```python
from build123d import *

# Parameters (mm, degrees)
SKETCH2_W             = 25
SKETCH2_H             = 25
BOSS_EXTRUDE1_DEPTH   = 760
BOSS_EXTRUDE1_2_DEPTH = 760
BOSS_EXTRUDE1_3_DEPTH = 760
BOSS_EXTRUDE1_4_DEPTH = 760
SKETCH3_W             = 25
SKETCH3_H             = 25
BOSS_EXTRUDE2_DEPTH   = 470
SKETCH6_W             = 25
SKETCH6_H             = 25
BOSS_EXTRUDE4_DEPTH   = 675
SKETCH10_W            = 25
SKETCH10_H            = 25
BOSS_EXTRUDE5_DEPTH   = 470
SKETCH11_W            = 25
SKETCH11_H            = 50
BOSS_EXTRUDE6_DEPTH   = 470
SKETCH12_R            = 650
BOSS_EXTRUDE7_DEPTH   = 20
SKETCH13_R            = 25
CUT_EXTRUDE3_DEPTH    = 20


with BuildPart() as part:
    # Sketch2 → Boss-Extrude1 (new body)
    with BuildSketch(Plane(origin=(0, 0, 0), x_dir=(1, 0, 0), z_dir=(0, 1, 0))):
        with Locations((-66.268467475, 428.678343046)):
            Rectangle(SKETCH2_W, SKETCH2_H)
    extrude(amount=-BOSS_EXTRUDE1_DEPTH)



with BuildPart() as body_2:
    # Sketch2 → Boss-Extrude1 2 (new body)
    with BuildSketch(Plane(origin=(0, 0, 0), x_dir=(1, 0, 0), z_dir=(0, 1, 0))):
        with Locations((628.731532525, 428.678343046)):
            Rectangle(SKETCH2_W, SKETCH2_H)
    extrude(amount=-BOSS_EXTRUDE1_2_DEPTH)


with BuildPart() as body_3:
    # Sketch2 → Boss-Extrude1 3 (new body)
    with BuildSketch(Plane(origin=(0, 0, 0), x_dir=(1, 0, 0), z_dir=(0, 1, 0))):
        with Locations((628.731532525, -61.321656954)):
            Rectangle(SKETCH2_W, SKETCH2_H)
    extrude(amount=-BOSS_EXTRUDE1_3_DEPTH)


with BuildPart() as body_4:
    # Sketch2 → Boss-Extrude1 4 (new body)
    with BuildSketch(Plane(origin=(0, 0, 0), x_dir=(1, 0, 0), z_dir=(0, 1, 0))):
        with Locations((-66.268467475, -61.321656954)):
            Rectangle(SKETCH2_W, SKETCH2_H)
    extrude(amount=-BOSS_EXTRUDE1_4_DEPTH)


with BuildPart() as part_1:
    add(part.part)

    add(body_2.part)  # Boss-Extrude2 merges body 2

    add(body_3.part)  # Boss-Extrude2 merges body 3

    add(body_4.part)  # Boss-Extrude2 merges body 4
    # Sketch3 → Boss-Extrude2 (add)
    with BuildSketch(Plane.XY.offset(-416.178343046)):
        with Locations((-66.268467475, -647.5)):
            Rectangle(SKETCH3_W, SKETCH3_H)
        with Locations((628.731532525, -647.5)):
            Rectangle(SKETCH3_W, SKETCH3_H)
    extrude(amount=BOSS_EXTRUDE2_DEPTH)

    # Sketch6 → Boss-Extrude4 (add)
    with BuildSketch(Plane(origin=(-53.768467475, 0, 0), x_dir=(0, 0, -1), z_dir=(1, 0, 0))):
        with Locations((428.678343046, -112.5)):
            Rectangle(SKETCH6_W, SKETCH6_H)
        with Locations((183.678343046, -647.5)):
            Rectangle(SKETCH6_W, SKETCH6_H)
        with Locations((-61.321656954, -112.5)):
            Rectangle(SKETCH6_W, SKETCH6_H)
    extrude(amount=BOSS_EXTRUDE4_DEPTH)

    # Sketch10 → Boss-Extrude5 (add)
    with BuildSketch(Plane(origin=(0, 0, 48.821656954), x_dir=(-1, 0, 0), z_dir=(0, 0, -1))):
        with Locations((-628.731532525, -112.5)):
            Rectangle(SKETCH10_W, SKETCH10_H)
        with Locations((66.268467475, -112.5)):
            Rectangle(SKETCH10_W, SKETCH10_H)
    extrude(amount=BOSS_EXTRUDE5_DEPTH)

    # Sketch11 → Boss-Extrude6 (add)
    with BuildSketch(Plane(origin=(0, 0, 48.821656954), x_dir=(-1, 0, 0), z_dir=(0, 0, -1))):
        with Locations((-628.731532525, -380.100970917)):
            Rectangle(SKETCH11_W, SKETCH11_H)
    extrude(amount=BOSS_EXTRUDE6_DEPTH)

    # Sketch12 → Boss-Extrude7 (add)
    with BuildSketch(Plane(origin=(0, 0, 0), x_dir=(1, 0, 0), z_dir=(0, 1, 0))):
        with Locations(Location((281.231532525, 183.678343046, 0), (0, 0, 270))):
            Circle(SKETCH12_R)
    extrude(amount=BOSS_EXTRUDE7_DEPTH)

    # Sketch13 → Cut-Extrude3 (cut)
    with BuildSketch(Plane(origin=(0, 0, 0), x_dir=(1, 0, 0), z_dir=(0, 1, 0))):
        with Locations(Location((281.231532525, 183.678343046, 0), (0, 0, 270))):
            Circle(SKETCH13_R)
    extrude(amount=CUT_EXTRUDE3_DEPTH, mode=Mode.SUBTRACT)


solid = part_1.part
```
Build history of the part. All positions in model axes, mm. A direction names the side the tool comes from. Coordinates: 2 decimals unless noted, no trailing zeros. Order: outer loops, then holes, each group sorted by start corner. A loop starts at its lowest first (then second) coordinate and runs counter-clockwise, first axis right, second up. Notation, with made-up numbers: (64.25, -16) -> (119.25, -16) arc R23 ccw to (119.25, 16) -> close; hole circle Ø8 at (65, -16.75). An arc over 180 degrees is marked (long way). Answer in a Markdown table with one row per item. Add a question column.
Q1. Wall check: line 1 along Y through (x, z) = (294, 305); line 2 along Z through (x, y) = (629, -110). Give the ranges that are in metal, low to high. Write a range as [from, to].
Q2. Band-saw the part on C-C, the plane z = -271. List the corners of the cut face in (x, y).
Q3. Band-saw the part on D-D, the plane z = -134. List the corners of the cut face in (x, y).
Q4. Which spindle directions (+Z, -Z, +X, -X, +Y, -Y) get a long thin tool onto all of the face, cutting with end or side? Do faces 4 (the face through (-53.768, -491, -419)), 5 (the face through (280, -635, -185)), 6 (the face through (259.052, 9.86, -172.142)), 7 (the face through (-53.768, -491, 51)). Say none if no direction does.
Q5. Drop flat-ended pins along their axis: pin 1 (4 mm diameter, centred on x = 502, z = -336, fed in from -Y); pin 2 (20 mm diameter, centred on x = -64.5, z = -258, fed in from -Y); pin 3 (7.5 mm diameter, centred on x = 631, y = -515.5, fed in from -Z). Give the stop position or say it passes through.
Q6. Band-saw the part on A-A, the plane y = -526. List the corners of the cut face in (x, z), then the cut area to 3 significant figures.
Q7. Band-saw the part on B-B, the plane x = 436.5. List the corners of the cut face in (y, z).
Q8. Mould opens along X. For faces 1 (the face through (279.6, -100.3, -441.178)), 2 (the face through (616.232, -397, -182)), 3 (the face through (-78.768, -354, 63)) say: +X half, -X half, draft (parallel to the pull), parting line (faces both ways), or undercut.
Answers follow:
| question | item | result |
|---|---|---|
| 1 | line 1 | [0, 20] |
| 1 | line 2 | [-441.18, 73.82] |
| 2 | outline | (-362.88, 0) -> (925.34, 0) -> (925.34, 20) -> (-362.88, 20) -> close; (-78.77, -660) -> (-53.77, -660) -> (-53.77, -635) -> (-78.77, -635) -> close; (-78.77, -125) -> (-53.77, -125) -> (-53.77, -100) -> (-78.77, -100) -> close; (616.23, -660) -> (641.23, -660) -> (641.23, -635) -> (616.23, -635) -> close; (616.23, -405.1) -> (641.23, -405.1) -> (641.23, -355.1) -> (616.23, -355.1) -> close; (616.23, -125) -> (641.23, -125) -> (641.23, -100) -> (616.23, -100) -> close |
| 3 | outline | (-366.87, 0) -> (929.33, 0) -> (929.33, 20) -> (-366.87, 20) -> close; (-78.77, -660) -> (-53.77, -660) -> (-53.77, -635) -> (-78.77, -635) -> close; (-78.77, -125) -> (-53.77, -125) -> (-53.77, -100) -> (-78.77, -100) -> close; (616.23, -660) -> (641.23, -660) -> (641.23, -635) -> (616.23, -635) -> close; (616.23, -405.1) -> (641.23, -405.1) -> (641.23, -355.1) -> (616.23, -355.1) -> close; (616.23, -125) -> (641.23, -125) -> (641.23, -100) -> (616.23, -100) -> close |
| 4 | face 4 | -Z, -Y |
| 4 | face 5 | +X, -X |
| 4 | face 6 | +Y |
| 4 | face 7 | +Z, -Y |
| 5 | pin 1 | y = 0 |
| 5 | pin 2 | y = -660 |
| 5 | pin 3 | z = -441.18 |
| 6 | outline | (-78.77, -441.18) -> (-53.77, -441.18) -> (-53.77, -416.18) -> (-78.77, -416.18) -> close; (-78.77, 48.82) -> (-53.77, 48.82) -> (-53.77, 73.82) -> (-78.77, 73.82) -> close; (616.23, -441.18) -> (641.23, -441.18) -> (641.23, -416.18) -> (616.23, -416.18) -> close; (616.23, 48.82) -> (641.23, 48.82) -> (641.23, 73.82) -> (616.23, 73.82) -> close |
| 6 | area | 2,500 mm^2 |
| 7 | outline | (-660, -196.18) -> (-635, -196.18) -> (-635, -171.18) -> (-660, -171.18) -> close; (-125, -441.18) -> (-100, -441.18) -> (-100, -416.18) -> (-125, -416.18) -> close; (-125, 48.82) -> (-100, 48.82) -> (-100, 73.82) -> (-125, 73.82) -> close; (0, -814.86) -> (20, -814.86) -> (20, 447.5) -> (0, 447.5) -> close |
| 8 | face 1 | draft |
| 8 | face 2 | undercut |
| 8 | face 3 | -X half |
